Geometry check sheet. Reference: the model listing, model coordinates, mm. Face numbers are marked on the shaded views. A direction names the side the tool comes from. Give positions to 0.01 mm unless a question says otherwise; leave off trailing zeros. Write each loop counter-clockwise with the first axis right and the second up, starting at its lowest first coordinate (ties: lowest second). Pieces come first, ordered by that corner, then holes. Notation, with made-up numbers: M 84.5,43 L 93.5,43 A15 cw 93.5,72 Z; hole C 38,70 d9. An arc over 180 degrees is marked long. Write each question's results on one line, items separated by ' | '.
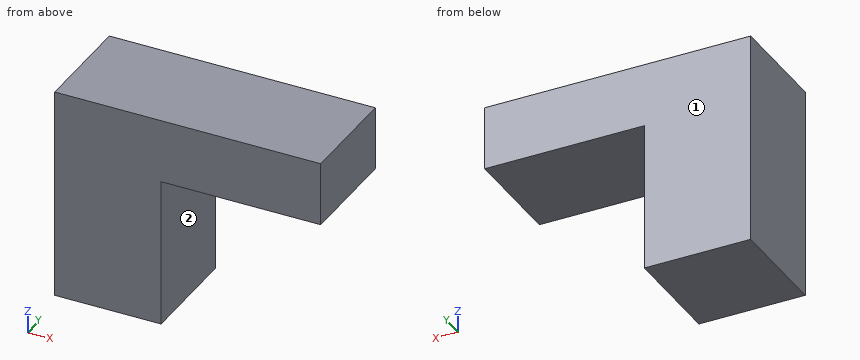
```python
from build123d import *

# Parameters (mm, degrees)
SCHIZZO1_W                   = 10
SCHIZZO1_H                   = 10
ESTRUSIONE_ESTRUSIONE1_DEPTH = 20
SCHIZZO2_W                   = 15
SCHIZZO2_H                   = 6
ESTRUSIONE_ESTRUSIONE2_DEPTH = 5


with BuildPart() as part:
    # Schizzo1 → Estrusione-Estrusione1 (new body)
    with BuildSketch(Plane.XY):
        Rectangle(SCHIZZO1_W, SCHIZZO1_H)
    extrude(amount=ESTRUSIONE_ESTRUSIONE1_DEPTH)

    # Schizzo2 → Estrusione-Estrusione2 (add, symmetric)
    with BuildSketch(Plane(origin=(0, 0, 0), x_dir=(1, 0, 0), z_dir=(0, 1, 0))):
        with Locations((12.5, -17)):
            Rectangle(SCHIZZO2_W, SCHIZZO2_H)
    extrude(amount=ESTRUSIONE_ESTRUSIONE2_DEPTH, both=True)


solid = part.part
```
Q1. Depth check by flat-ended pin: P1, Ø5, axis at y = -2, z = 5, coming from the +X side; P2, Ø3, axis at x = 14.5, y = 2.5, coming from the -Z side. Enter the tip coordinate at first touch or a pass-through.
Answer key:
P1: stops at x = 5 | P2: stops at z = 14
Q2. Section check A-A (y = -2.75). Enter the section's corners in (x, z).
Answer key:
outline: M -5,0 L 5,0 L 5,14 L 20,14 L 20,20 L -5,20 Z
Q3. Access from +Z, -Z, +X, -X, +Y, -Y to the whole of each face (thin tool, end or side, straight path). Record for the marked faces 1 and 2.
Answer key:
face 1: +Z, -Z, +X, -X, +Y | face 2: -Z, +X, +Y, -Y
Q4. Section check B-B (x = 10.5). Enter the section's corners in (y, z), then the cut area to 3 significant figures.
Answer key:
outline: M -5,14 L 5,14 L 5,20 L -5,20 Z | area: 60.0 mm2
Q5. Material ranges on probe 1 along X at (y, z) = (4.5, 2.5); probe 2 along Z at (x, y) = (18.5, -1.25), recorded low to high. Write a range as [from, to].
Answer key:
probe 1: x = [-5, 5] | probe 2: z = [14, 20]
Q6. Section check C-C (z = 5.25). Enter the section's corners in (x, y).
Answer key:
outline: M -5,-5 L 5,-5 L 5,5 L -5,5 Z
